Check sheet for the modelled part. Datum: model origin and axes. Units: mm. Face numbers are marked on the shaded views. A direction names the side the tool comes from. Coordinates: 2 decimals unless noted, no trailing zeros. Write each loop counter-clockwise with the first axis right and the second up, starting at its lowest first coordinate (ties: lowest second). Pieces come first, ordered by that corner, then holes. Notation, with made-up numbers: (-3.75, -20.5) -> (55.25, -20.5) arc R20 cw to (55.25, 18.5) -> close; hole circle Ø7 at (-26, -37). An arc over 180 degrees is marked (long way). Put each result on its own line as item: value.
```python
from build123d import *

# Parameters (mm, degrees)
SKETCH_1_W          = 250
SKETCH_1_H          = 250
EXTRUDE_1_DEPTH     = 180
CHAMFER_1_SIZE      = 50
CHAMFER_1_SIZE2     = 86.602540378
SKETCH_2_R          = 27.5
EXTRUDE_2_DEPTH     = 20
EXTRUDE_START       = 20
SKETCH_2_3_R        = 32.5
SKETCH_2_3_R_2      = 27.5
EXTRUDE_3_DEPTH     = 8
FILLET_1_R          = 10
CUT_EXTRUDE_START   = -10
CUT_EXTRUDE_1_DEPTH = 230


with BuildPart() as part:
    # Sketch 1 → Extrude 1 (new body)
    with BuildSketch(Plane(origin=(0, 0, 0), x_dir=(1, 0, 0), z_dir=(0, 1, 0))):
        with Locations((125, 125)):
            Rectangle(SKETCH_1_W, SKETCH_1_H)
    extrude(amount=EXTRUDE_1_DEPTH)

    # Chamfer 1
    chamfer_1_edges = [part.edges().sort_by_distance(p)[0] for p in [
        (125, 180, 0),
    ]]
    chamfer_1_side = [part.faces().sort_by_distance(p)[0] for p in [
        (125, 90, 0),
    ]]
    chamfer(chamfer_1_edges, length=CHAMFER_1_SIZE, length2=CHAMFER_1_SIZE2, reference=chamfer_1_side[0])

    # Sketch 2 → Extrude 2 (add)
    with BuildSketch(Plane(origin=(0, 97.5, 56.291651246), x_dir=(1, 0, 0), z_dir=(0, 0.866025404, 0.5))):
        with Locations((125, 115)):
            Circle(SKETCH_2_R)
    extrude(amount=EXTRUDE_2_DEPTH)

    # Sketch 2_3 → Extrude 3 (add)
    with BuildSketch(Plane(origin=(0, 97.5, 56.291651246), x_dir=(1, 0, 0), z_dir=(0, 0.866025404, 0.5)).offset(EXTRUDE_START)):
        with Locations((125, 115)):
            Circle(SKETCH_2_3_R)
        with Locations((125, 115)):
            Circle(SKETCH_2_3_R_2, mode=Mode.SUBTRACT)
    extrude(amount=-EXTRUDE_3_DEPTH)

    # Fillet 1
    fillet_1_edges = [part.edges().sort_by_distance(p)[0] for p in [
        (125, 180, -250),
        (250, 180, -168.301270189),
        (125, 180, -86.602540378),
        (250, 65, 0),
        (250, 155, -43.301270189),
        (0, 65, 0),
        (125, 130, 0),
        (0, 155, -43.301270189),
        (97.5, 155, -43.301270189),
        (0, 180, -168.301270189),
        (125, 0, -250),
        (250, 0, -125),
        (125, 0, 0),
        (0, 0, -125),
        (0, 90, -250),
        (250, 90, -250),
    ]]
    fillet(fillet_1_edges, radius=FILLET_1_R)

    # Sketch 3 → Cut-Extrude 1 (cut)
    with BuildSketch(Plane(origin=(250, 0, 0), x_dir=(0, 0, -1), z_dir=(1, 0, 0)).offset(CUT_EXTRUDE_START)):
        Polygon((237, 13), (237, 167), (90.08587988, 167), (13, 122.494446501), (13, 13), align=None)
    extrude(amount=-CUT_EXTRUDE_1_DEPTH, mode=Mode.SUBTRACT)


solid = part.part
```
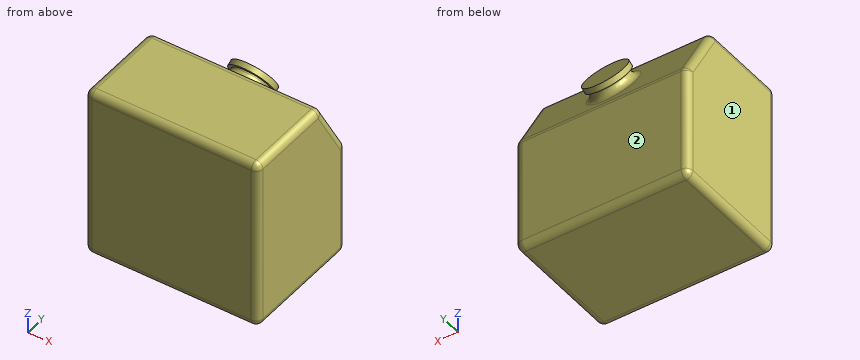
Q1. Tool access check on the marked faces 1 and 2. Record the directions out of +Z, -Z, +X, -X, +Y, -Y that give a thin tool (end or side, any length) a straight path to the whole face; none if there is none.
Recorded:
face 1: +Z, -Z, -X, +Y, -Y
face 2: -Z, +X, -X, +Y
Q2. Cross-section at C-C (z = -216). Record the cut outline in (x, y), plus the area to 3 significant figures.
Recorded:
outline: (0, 10) arc R10 ccw to (10, 0) -> (240, 0) arc R10 ccw to (250, 10) -> (250, 170) arc R10 ccw to (240, 180) -> (10, 180) arc R10 ccw to (0, 170) -> close; hole (10, 13) -> (240, 13) -> (240, 167) -> (10, 167) -> close
area: 9,490 mm2
Q3. Material ranges on line 1 along X through (y, z) = (137, -56); line 2 along Y through (x, z) = (171.5, -95.5); line 3 along Z through (x, y) = (17, 52.5), recorded low to high.
Recorded:
line 1: x = 0 to 10, 240 to 250
line 2: y = 0 to 13, 167 to 180
line 3: z = -250 to -237, -13 to 0
Q4. Cross-section at A-A (x = 63). Record the cut outline in (y, z), plus the area to 3 significant figures.
Recorded:
outline: (0, -240) arc R10 ccw to (10, -250) -> (170, -250) arc R10 ccw to (180, -240) -> (180, -89.28) arc R10 ccw to (178.66, -84.28) -> (132.89, -5) arc R10 ccw to (124.23, 0) -> (10, 0) arc R10 ccw to (0, -10) -> close; hole (13, -237) -> (167, -237) -> (167, -90.09) -> (122.49, -13) -> (13, -13) -> close
area: 9,980 mm2
Q5. Depth check by flat-ended pin: P1, Ø4, axis at x = 34.5, y = 127, coming from the +Z side; P2, Ø12, axis at x = 96, z = -141, coming from the +Y side; P3, Ø2, axis at x = 221.5, z = -49.5, coming from the +Y side. Enter the tip coordinate at first touch or a pass-through.
Recorded:
P1: stops at z = -0.03
P2: stops at y = 180
P3: stops at y = 159.16
Q6. Cross-section at B-B (y = 84). Record the cut outline in (x, z).
Recorded:
outline: (0, -240) arc R10 ccw to (10, -250) -> (240, -250) arc R10 ccw to (250, -240) -> (250, -10) arc R10 ccw to (240, 0) -> (10, 0) arc R10 ccw to (0, -10) -> close; hole (10, -237) -> (240, -237) -> (240, -13) -> (10, -13) -> close
